from build123d import *

# Parameters (mm, degrees)
PLATE_MAIN_SKETCH_R            = 0.86491532
PLATE_MAIN_SKETCH_R_2          = 8.982669203
PLATE_MAIN_SKETCH_R_3          = 2.111650326
EXTRUDE_PLATE_MAIN_DEPTH       = 4
CBORE_FOR_M3_SHCS1_AT_2_COUNT  = 2
CBORE_FOR_M3_SHCS1_AT_2_PITCH  = 31
CBORE_FOR_M3_SHCS1_AT_3_COUNT  = 2
CBORE_FOR_M3_SHCS1_AT_3_PITCH  = 43.840620434
CBORE_FOR_M3_SHCS1_AT_4_COUNT  = 2
CBORE_FOR_M3_SHCS1_AT_4_PITCH  = 31
CBORE_FOR_M3_SHCS1_AT_5_COUNT  = 2
CBORE_FOR_M3_SHCS1_AT_5_PITCH  = 41.615227408
CBORE_FOR_M3_SHCS1_AT_6_COUNT  = 2
CBORE_FOR_M3_SHCS1_AT_6_PITCH  = 51.800096525
CBORE_FOR_M3_SHCS1_AT_7_COUNT  = 2
CBORE_FOR_M3_SHCS1_AT_7_PITCH  = 67.091355628
CBORE_FOR_M3_SHCS1_AT_8_COUNT  = 2
CBORE_FOR_M3_SHCS1_AT_8_PITCH  = 59.580425915
CBORE_FOR_M3_SHCS1_AT_9_COUNT  = 2
CBORE_FOR_M3_SHCS1_AT_9_PITCH  = 101.688249075
CBORE_FOR_M3_SHCS1_AT_10_COUNT = 2
CBORE_FOR_M3_SHCS1_AT_10_PITCH = 111.581808553


with BuildPart() as part:
    # Plate Main Sketch → Extrude Plate Main (new body)
    with BuildSketch(Plane(origin=(-158.085545862, 0, 24.679095537), x_dir=(-1, 0, 0), z_dir=(0, 1, 0))):
        with BuildLine():
            Line((-178.585545862, -24.679095537), (-137.585545862, -24.679095537))
            Line((-137.585545862, -24.679095537), (-137.585545862, -12.679095537))
            ThreePointArc((-137.585545862, -12.679095537), (-136.121079768, -9.143561631), (-132.585545862, -7.679095537))
            Line((-132.585545862, -7.679095537), (-129.585545862, -7.679095537))
            Line((-129.585545862, -7.679095537), (-129.585545862, 54.820904463))
            ThreePointArc((-129.585545862, 54.820904463), (-128.853312815, 56.588671416), (-127.085545862, 57.320904463))
            Line((-127.085545862, 57.320904463), (-127.085545862, 83.320904463))
            ThreePointArc((-127.085545862, 83.320904463), (-128.853312815, 84.05313751), (-129.585545862, 85.820904463))
            Line((-129.585545862, 85.820904463), (-129.585545862, 101.320904463))
            Line((-129.585545862, 101.320904463), (-186.585545862, 101.320904463))
            Line((-186.585545862, 101.320904463), (-186.585545862, 85.820904463))
            ThreePointArc((-186.585545862, 85.820904463), (-187.317778909, 84.05313751), (-189.085545862, 83.320904463))
            Line((-189.085545862, 83.320904463), (-189.085545862, 57.320904463))
            ThreePointArc((-189.085545862, 57.320904463), (-187.317778909, 56.588671416), (-186.585545862, 54.820904463))
            Line((-186.585545862, 54.820904463), (-186.585545862, -7.679095537))
            Line((-186.585545862, -7.679095537), (-183.585545862, -7.679095537))
            ThreePointArc((-183.585545862, -7.679095537), (-180.050011956, -9.143561631), (-178.585545862, -12.679095537))
            Line((-178.585545862, -12.679095537), (-178.585545862, -24.679095537))
        make_face()
        with Locations(Location((-134.585545862, 96.820904463, 0), (0, 0, 90))):
            Circle(PLATE_MAIN_SKETCH_R, mode=Mode.SUBTRACT)
        with Locations(Location((-134.585545862, 64.820904463, 0), (0, 0, 90))):
            Circle(PLATE_MAIN_SKETCH_R, mode=Mode.SUBTRACT)
        with Locations(Location((-181.585545862, 64.820904463, 0), (0, 0, 90))):
            Circle(PLATE_MAIN_SKETCH_R, mode=Mode.SUBTRACT)
        with Locations(Location((-181.585545862, 96.820904463, 0), (0, 0, 90))):
            Circle(PLATE_MAIN_SKETCH_R, mode=Mode.SUBTRACT)
        with Locations(Location((-170.241643156, -16.679095537, 0), (0, 0, 90))):
            Circle(PLATE_MAIN_SKETCH_R, mode=Mode.SUBTRACT)
        with Locations(Location((-170.241643156, 3.320904463, 0), (0, 0, 90))):
            Circle(PLATE_MAIN_SKETCH_R, mode=Mode.SUBTRACT)
        with Locations(Location((-170.241643156, 23.320904463, 0), (0, 0, 90))):
            Circle(PLATE_MAIN_SKETCH_R, mode=Mode.SUBTRACT)
        with Locations(Location((-170.241643156, 43.320904463, 0), (0, 0, 90))):
            Circle(PLATE_MAIN_SKETCH_R, mode=Mode.SUBTRACT)
        with Locations(Location((-145.929448569, -16.679095537, 0), (0, 0, 270))):
            Circle(PLATE_MAIN_SKETCH_R, mode=Mode.SUBTRACT)
        with Locations(Location((-145.929448569, 3.320904463, 0), (0, 0, 270))):
            Circle(PLATE_MAIN_SKETCH_R, mode=Mode.SUBTRACT)
        with Locations(Location((-145.929448569, 23.320904463, 0), (0, 0, 270))):
            Circle(PLATE_MAIN_SKETCH_R, mode=Mode.SUBTRACT)
        with Locations(Location((-145.929448569, 43.320904463, 0), (0, 0, 270))):
            Circle(PLATE_MAIN_SKETCH_R, mode=Mode.SUBTRACT)
        with Locations(Location((-158.085545862, 80.320904463, 0), (0, 0, 90))):
            Circle(PLATE_MAIN_SKETCH_R_2, mode=Mode.SUBTRACT)
        with Locations(Location((-158.085545862, 55.320904463, 0), (0, 0, 90))):
            Circle(PLATE_MAIN_SKETCH_R_3, mode=Mode.SUBTRACT)
    extrude(amount=EXTRUDE_PLATE_MAIN_DEPTH)

    # Sketch5 → CBORE for M3 SHCS1 (revolve, cut)
    with BuildSketch(Plane(origin=(-15.5, 0, 120.5), x_dir=(0, 0, -1), z_dir=(1, 0, 0))):
        Polygon((0, 0), (0, 4), (1.725, 4), (1.7, 3.975), (1.7, 3), (3, 3), (3, 0), align=None)
    cbore_for_m3_shcs1 = revolve(axis=Axis((-15.5, -6.35, 120.5), (0, 1, 0)), mode=Mode.SUBTRACT)

    # CBORE for M3 SHCS1 at 2: CBORE for M3 SHCS1 ×2
    with Locations(*[(i * CBORE_FOR_M3_SHCS1_AT_2_PITCH, 0, 0) for i in range(1, CBORE_FOR_M3_SHCS1_AT_2_COUNT)]):
        add(cbore_for_m3_shcs1, mode=Mode.SUBTRACT)

    # CBORE for M3 SHCS1 at 3: CBORE for M3 SHCS1 ×2
    with Locations(*[Vector(0.7071067811865482, 0, -0.7071067811865469) * (i * CBORE_FOR_M3_SHCS1_AT_3_PITCH) for i in range(1, CBORE_FOR_M3_SHCS1_AT_3_COUNT)]):
        add(cbore_for_m3_shcs1, mode=Mode.SUBTRACT)

    # CBORE for M3 SHCS1 at 4: CBORE for M3 SHCS1 ×2
    with Locations(*[(0, 0, -i * CBORE_FOR_M3_SHCS1_AT_4_PITCH) for i in range(1, CBORE_FOR_M3_SHCS1_AT_4_COUNT)]):
        add(cbore_for_m3_shcs1, mode=Mode.SUBTRACT)

    # CBORE for M3 SHCS1 at 5: CBORE for M3 SHCS1 ×2
    with Locations(*[Vector(-0.07436454462395926, 0, -0.9972311239140459) * (i * CBORE_FOR_M3_SHCS1_AT_5_PITCH) for i in range(1, CBORE_FOR_M3_SHCS1_AT_5_COUNT)]):
        add(cbore_for_m3_shcs1, mode=Mode.SUBTRACT)

    # CBORE for M3 SHCS1 at 6: CBORE for M3 SHCS1 ×2
    with Locations(*[Vector(0.5984544832852718, 0, -0.801156808268992) * (i * CBORE_FOR_M3_SHCS1_AT_6_PITCH) for i in range(1, CBORE_FOR_M3_SHCS1_AT_6_COUNT)]):
        add(cbore_for_m3_shcs1, mode=Mode.SUBTRACT)

    # CBORE for M3 SHCS1 at 7: CBORE for M3 SHCS1 ×2
    with Locations(*[Vector(0.4620565452857235, 0, -0.8868504659516295) * (i * CBORE_FOR_M3_SHCS1_AT_7_PITCH) for i in range(1, CBORE_FOR_M3_SHCS1_AT_7_COUNT)]):
        add(cbore_for_m3_shcs1, mode=Mode.SUBTRACT)

    # CBORE for M3 SHCS1 at 8: CBORE for M3 SHCS1 ×2
    with Locations(*[Vector(-0.051941512469712944, 0, -0.9986501285647335) * (i * CBORE_FOR_M3_SHCS1_AT_8_PITCH) for i in range(1, CBORE_FOR_M3_SHCS1_AT_8_COUNT)]):
        add(cbore_for_m3_shcs1, mode=Mode.SUBTRACT)

    # CBORE for M3 SHCS1 at 9: CBORE for M3 SHCS1 ×2
    with Locations(*[Vector(0.15242665834989946, 0, -0.9883147847848291) * (i * CBORE_FOR_M3_SHCS1_AT_9_PITCH) for i in range(1, CBORE_FOR_M3_SHCS1_AT_9_COUNT)]):
        add(cbore_for_m3_shcs1, mode=Mode.SUBTRACT)

    # CBORE for M3 SHCS1 at 10: CBORE for M3 SHCS1 ×2
    with Locations(*[Vector(0.13891153227375588, 0, -0.9903047945967732) * (i * CBORE_FOR_M3_SHCS1_AT_10_PITCH) for i in range(1, CBORE_FOR_M3_SHCS1_AT_10_COUNT)]):
        add(cbore_for_m3_shcs1, mode=Mode.SUBTRACT)


solid = part.part
Part model, mm, in its own coordinate system. A direction names the side the tool comes from. Give positions to 0.01 mm unless a question says otherwise; leave off trailing zeros. Loops run counter-clockwise (first coordinate to the right, second up) from the corner with the lowest first, then second, coordinate; pieces in that order, holes last. Notation, with made-up numbers: M 8,51 L 42,51 A27 cw 42,75 Z; hole C 72.25,-25 d3. An arc over 180 degrees is marked long. Put each result on its own line as item: value. Start each with the question number.
1) 3-axis set-ups, long thin cutter, end or side, ignore diameter. For faces 5 (the flat face through (-28.5, 2, 48)), 6 (the cylindrical face through (-0.81, 1.97, 81.95)), 7 (the cylindrical face through (-14.35, 1.48, 117.73)): which of +Z, -Z, +X, -X, +Y, -Y reach the whole face in a straight line?
2) Pull direction Z, two halves, no side cores. Call faces 1 (the flat face through (0, 0, 64)), 2 (the flat face through (0, 2, 126)), 3 (the flat face through (17.5, 3, 79)), 4 (the cylindrical face through (-29, 2, 81)): +Z half, -Z half, draft (parallel to the pull), parting line (faces both ways), or undercut.
3) Probe probe 1 along X at (y, z) = (3.6, 61); probe 2 along Z at (x, y) = (-15.5, 1.3); probe 3 along X at (y, z) = (3.65, 79). List the from-to ranges inside material, lowest first.
4) Saw through at B-B (x = 0). State how many separate pieces and enclosed holes the cut face has, then the cut area to 3 significant figures.
5) Saw through at A-A (z = 10). List the corners of the cut face in (x, y) (3 decimals), then the cut area to 3 significant figures.
6) Flat gauge pins, fed straight in: pin 1 (3 mm diameter, centred on x = -23.5, z = 121.5, fed in from -Y); pin 2 (2 mm diameter, centred on y = 3, z = 6.5, fed in from +X); pin 3 (1.5 mm diameter, centred on y = 1.5, z = 23.5, fed in from -X); pin 4 (4 mm diameter, centred on x = -15.5, z = 89.5, fed in from -Y). Where does each tip first touch, or does it go through?
7) Saw through at C-C (z = 50). List the corners of the cut face in (x, y).
Numbers:
1. face 5: -Z, -X, +Y, -Y
1. face 6: +Y, -Y
1. face 7: -Y
2. face 1: draft
2. face 2: +Z half
2. face 3: undercut
2. face 4: -Z half
3. probe 1: -28.5 to -20.29, -16.89 to 13.8, 17.2 to 28.5
3. probe 2: 0 to 86.5, 92.5 to 117.5, 123.5 to 126
3. probe 3: -28.5 to -20.29, -16.89 to -1.86, 1.86 to 13.8, 17.2 to 28.5
4. separate pieces: 5
4. enclosed holes: 0
4. area: 372 mm^2
5. outline: M -20.5,0 L -3,0 L -3,3 L -1.7,3 L -1.7,3.975 L -1.725,4 L -20.5,4 Z; M 1.7,3 L 3,3 L 3,0 L 20.5,0 L 20.5,4 L 1.725,4 L 1.7,3.975 Z
5. area: 143 mm^2
6. pin 1: y = 0
6. pin 2: x = 20.5
6. pin 3: x = -28.5
6. pin 4: y = 3
7. outline: M -28.5,0 L 28.5,0 L 28.5,4 L -28.5,4 Z
